Autodesk Inventor part; units mm, degrees
ref_plane "C1_XY" through (0, 0, 0) normal (0, 0, 1) x (1, 0, 0)
ref_plane "C1_YZ" through (0, 0, 0) normal (1, 0, 0) x (0, 1, 0)
ref_plane "C1_ZX" through (0, 0, 0) normal (0, 1, 0) x (0, 0, 1)
sketch "Sketch_1" plane through (0, 0, 0) normal (0, 0, 1) x (1, 0, 0)
  line L0 (-15, -4) -> (-15, -13)
  arc A0 (-15, -13) -> (-13, -15) centre (-13, -13) ccw
  line L1 (-13, -15) -> (-4, -15)
  line L2 (-4, -15) -> (-4, -13)
  line L3 (-4, -13) -> (-8.25, -13)
  line L4 (-8.25, -13) -> (-8.25, -9.6642)
  line L5 (-8.25, -9.6642) -> (-4.5858, -6)
  line L6 (-4.5858, -6) -> (-0.5196, -6)
  line L7 (-0.5196, -6) -> (0, -5.7)
  line L8 (0, -5.7) -> (0.5196, -6)
  line L9 (0.5196, -6) -> (4.5858, -6)
  line L10 (4.5858, -6) -> (8.25, -9.6642)
  line L11 (8.25, -9.6642) -> (8.25, -13)
  line L12 (8.25, -13) -> (4, -13)
  line L13 (4, -13) -> (4, -15)
  line L14 (4, -15) -> (13, -15)
  arc A1 (13, -15) -> (15, -13) centre (13, -13) ccw
  line L15 (15, -13) -> (15, -4)
  line L16 (15, -4) -> (13, -4)
  line L17 (13, -4) -> (13, -8.25)
  line L18 (13, -8.25) -> (9.6642, -8.25)
  line L19 (9.6642, -8.25) -> (6, -4.5858)
  line L20 (6, -4.5858) -> (6, -0.5196)
  line L21 (6, -0.5196) -> (5.7, 0)
  line L22 (5.7, 0) -> (6, 0.5196)
  line L23 (6, 0.5196) -> (6, 4.5858)
  line L24 (6, 4.5858) -> (9.6642, 8.25)
  line L25 (9.6642, 8.25) -> (13, 8.25)
  line L26 (13, 8.25) -> (13, 4)
  line L27 (13, 4) -> (15, 4)
  line L28 (15, 4) -> (15, 13)
  arc A2 (15, 13) -> (13, 15) centre (13, 13) ccw
  line L29 (13, 15) -> (4, 15)
  line L30 (4, 15) -> (4, 13)
  line L31 (4, 13) -> (8.25, 13)
  line L32 (8.25, 13) -> (8.25, 9.6642)
  line L33 (8.25, 9.6642) -> (4.5858, 6)
  line L34 (4.5858, 6) -> (0.5196, 6)
  line L35 (0.5196, 6) -> (0, 5.7)
  line L36 (0, 5.7) -> (-0.5196, 6)
  line L37 (-0.5196, 6) -> (-4.5858, 6)
  line L38 (-4.5858, 6) -> (-8.25, 9.6642)
  line L39 (-8.25, 9.6642) -> (-8.25, 13)
  line L40 (-8.25, 13) -> (-4, 13)
  line L41 (-4, 13) -> (-4, 15)
  line L42 (-4, 15) -> (-13, 15)
  arc A3 (-13, 15) -> (-15, 13) centre (-13, 13) ccw
  line L43 (-15, 13) -> (-15, 4)
  line L44 (-15, 4) -> (-13, 4)
  line L45 (-13, 4) -> (-13, 8.25)
  line L46 (-13, 8.25) -> (-9.6642, 8.25)
  line L47 (-9.6642, 8.25) -> (-6, 4.5858)
  line L48 (-6, 4.5858) -> (-6, 0.5196)
  line L49 (-6, 0.5196) -> (-5.7, 0)
  line L50 (-5.7, 0) -> (-6, -0.5196)
  line L51 (-6, -0.5196) -> (-6, -4.5858)
  line L52 (-6, -4.5858) -> (-9.6642, -8.25)
  line L53 (-9.6642, -8.25) -> (-13, -8.25)
  line L54 (-13, -8.25) -> (-13, -4)
  line L55 (-13, -4) -> (-15, -4)
extrude "Extrusion1" add sketch "Sketch_1" against normal blind 1005.5
sketch "Sketch2" plane through (0, 0, -1005.5) normal (0, 0, -1) x (-1, 0, 0)
  point P0 (0, 0)
hole "Hole1" at (0, 0, -1005.5) direction (0, 0, 1) diameter 6.8 depth 1005.5
sketch "Sketch3" plane through (0, 0, -1005.5) normal (0, 0, -1) x (-1, 0, 0)
  point P0 (-11.6, 11.6)
hole "Hole2" at (11.6, 11.6, -1005.5) direction (0, 0, 1) diameter 4.2 depth 1005.5
pattern_linear "Rectangular Pattern1" count 2 spacing 23.2 along (-1, 0, 0) count 2 spacing 23.2 along (0, -1, 0) of "Hole2"
sketch "Sketch_5" plane through (0, 0, 0) normal (1, 0, 0) x (0, 0, -1)
  line L0 (0, 15) -> (0, -15)
  line L1 (0, -15) -> (30, -15)
  line L2 (30, -15) -> (0, 15)
extrude "Extrusion2" cut sketch "Sketch_5" along normal mid plane 30
sketch "Sketch_8" plane through (0, 0, 0) normal (1, 0, 0) x (0, 0, -1)
  line L0 (975.5, 15) -> (1005.5, -15)
  line L1 (1005.5, -15) -> (1005.5, 15)
  line L2 (1005.5, 15) -> (975.5, 15)
extrude "Extrusion3" cut sketch "Sketch_8" along normal mid plane 30
ref_plane "C1_XY" through (0, 0, 0) normal (0, 0, 1) x (1, 0, 0)
ref_plane "C1_YZ" through (0, 0, 0) normal (1, 0, 0) x (0, 1, 0)
ref_plane "C1_ZX" through (0, 0, 0) normal (0, 1, 0) x (0, 0, 1)
ref_plane "to_frame_cap1_XY" through (0, 0, 0) normal (0, 0, 1) x (1, 0, 0)
ref_plane "to_frame_cap1_YZ" through (0, 0, 0) normal (1, 0, 0) x (0, 1, 0)
ref_plane "to_frame_cap1_ZX" through (0, 0, 0) normal (0, 1, 0) x (0, 0, 1)
ref_plane "to_frame_cap2_XY" through (0, 0, -1005.5) normal (0, 0, -1) x (1, 0, 0)
ref_plane "to_frame_cap2_YZ" through (0, 0, -1005.5) normal (1, 0, 0) x (0, -1, 0)
ref_plane "to_frame_cap2_ZX" through (0, 0, -1005.5) normal (0, -1, 0) x (0, 0, -1)
properties part number "HFS6-3030-1005.5-LAT45-RCT45"
Geometry check sheet. Reference: the model listing, model coordinates, mm. Give positions to 0.01 mm unless a question says otherwise; leave off trailing zeros.
1) Gauge pin test, flat ends, axial feed: pin 1 (8 mm diameter, centred on x = 7, y = -7, fed in from -Z); pin 2 (2.5 mm diameter, centred on x = 11.6, y = 11.6, fed in from -Z); pin 3 (1.2 mm diameter, centred on x = -3.5, z = -522.5, fed in from -Y); pin 4 (1.6 mm diameter, centred on y = 14, z = -481, fed in from +X). Record the tip position at first contact, or that the pin passes through.
2) Section check A-A, the plane z = -325. State how many separate pieces and enclosed holes the cut face has, and give its area (3 significant figures).
3) Material ranges on L1, parallel to Y at x = -12.25, z = -551; L2, parallel to Y at x = -11.6, z = -667; L3, parallel to X at y = -12, z = -535.5, recorded low to high.
Computed:
1. pin 1: stops at z = -1001.3
1. pin 2: passes through
1. pin 3: stops at y = -15
1. pin 4: stops at x = 14.99
2. separate pieces: 1
2. enclosed holes: 5
2. area: 332 mm2
3. L1: y = -15 to -13.6, -9.6 to -8.25, 8.25 to 9.6, 13.6 to 15
3. L2: y = -15 to -13.7, -9.5 to -8.25, 8.25 to 9.5, 13.7 to 15
3. L3: x = -15 to -13.66, -9.54 to -8.25, 8.25 to 9.54, 13.66 to 15
